Geometry: final body of the model. Coordinates: model frame, mm. A direction names the side the tool comes from. Give positions to 0.01 mm unless a question says otherwise; leave off trailing zeros. Loops run counter-clockwise (first coordinate to the right, second up) from the corner with the lowest first, then second, coordinate; pieces in that order, holes last. Notation, with made-up numbers: (-36, -26) -> (-20, -26) arc R23 cw to (-20, -5) -> close; hole circle Ø6 at (-28.75, 86). An arc over 180 degrees is marked (long way). One line per item, written item: value. Start each with the question number.
from build123d import *

# Parameters (mm, degrees)
F_4_5_4_5_DIAMETER_HOLE1_D = 4.5
CIRPATTERN1_COUNT          = 12
F_4_0_4_DIAMETER_HOLE1_D   = 4
CIRPATTERN2_COUNT          = 4
CIRPATTERN3_COUNT          = 4


with BuildPart() as part:
    # Sketch1 → Revolve1 (revolve)
    with BuildSketch(Plane(origin=(0, 0, 0), x_dir=(0, 0, -1), z_dir=(1, 0, 0)), mode=Mode.PRIVATE) as revolve1_sk:
        with BuildLine():
            Line((0, 129), (0, 121.95))
            ThreePointArc((0, 121.95), (-0.878679656, 119.828679656), (-3, 118.95))
            Line((-3, 118.95), (-28, 118.95))
            Line((-28, 118.95), (-28, 119.95))
            Line((-28, 119.95), (-3, 119.95))
            ThreePointArc((-3, 119.95), (-1.585786438, 120.535786438), (-1, 121.95))
            Line((-1, 121.95), (-1, 129))
            Line((-1, 129), (0, 129))
        make_face()
    revolve(revolve1_sk.sketch.rotate(Axis((0, 0, 36.289125048), (0, 0, -1)), 90), axis=Axis((0, 0, 36.289125048), (0, 0, -1)))  # turned: the seam where the file's is

    # Ø4.5 (4.5) Diameter Hole1 (through all)
    with Locations(Plane.XY.offset(1)):
        with Locations((62.125, 107.60365642)):
            f_4_5_4_5_diameter_hole1 = Hole(F_4_5_4_5_DIAMETER_HOLE1_D / 2)

    # CirPattern1: Ø4.5 (4.5) Diameter Hole1 ×12 about axis, 4 skipped
    cirpattern1_axis = Axis((0, 0, -80.9), (0, 0, 1))
    add([f_4_5_4_5_diameter_hole1.rotate(cirpattern1_axis, i * 360 / CIRPATTERN1_COUNT) for i in range(1, CIRPATTERN1_COUNT) if i not in (1, 4, 7, 10)], mode=Mode.SUBTRACT)

    # Ø4.0 (4) Diameter Hole1 (through all)
    with Locations(Plane.XY.offset(1)):
        with Locations((124.25, 0)):
            f_4_0_4_diameter_hole1 = Hole(F_4_0_4_DIAMETER_HOLE1_D / 2)

    # CirPattern2: Ø4.0 (4) Diameter Hole1 ×4 about axis
    cirpattern2_axis = Axis((0, 0, 0), (0, 0, 1))
    for i in range(1, CIRPATTERN2_COUNT):
        add(f_4_0_4_diameter_hole1.rotate(cirpattern2_axis, i * 360 / CIRPATTERN2_COUNT), mode=Mode.SUBTRACT)

    # Sketch7 → Ø4.5 (4.5) Diameter Hole2 (revolve, cut)
    with BuildSketch(Plane(origin=(87.858017562, 87.858017562, 1), x_dir=(0, -1, 0), z_dir=(1, 0, 0))):
        Polygon((0, 0), (0, 2.851936393), (2.25, 1.5), (2.25, 0), align=None)
    f_4_5_4_5_diameter_hole2 = revolve(axis=Axis((87.858017562, 87.858017562, 7.35), (0, 0, -1)), mode=Mode.SUBTRACT)

    # CirPattern3: Ø4.5 (4.5) Diameter Hole2 ×4 about axis
    cirpattern3_axis = Axis((0, 0, 0), (0, 0, 1))
    for i in range(1, CIRPATTERN3_COUNT):
        add(f_4_5_4_5_diameter_hole2.rotate(cirpattern3_axis, i * 360 / CIRPATTERN3_COUNT), mode=Mode.SUBTRACT)


solid = part.part
Item 1: Pin query (flat end, axial travel): pin 1 (6 mm diameter, centred on y = 17.5, z = 10.5, fed in from -X); pin 2 (6 mm diameter, centred on x = 87.86, y = -87.86, fed in from +Z); pin 3 (3.5 mm diameter, centred on x = -62.12, y = 107.6, fed in from +Z); pin 4 (4 mm diameter, centred on x = -82.5, z = 25, fed in from +Y). Return the tip coordinate at first contact, or that it passes through.
Item 2: Mould query, pull axis Y, two halves, no side actions, for faces 3 (the face through (113.457, -35.729, 15.675)), 4 (the face through (123.043, -38.748, 0.493)), 5 (the face through (116, -27, 28)). Classes: pulls with the +Y half, pulls with the -Y half, needs draft (parallel to the pull), parting line crosses it, or undercut.
Item 3: Ray query, line 1 along X through (y, z) = (-68, 26); line 2 along Y through (x, z) = (66.5, 6); line 3 along Y through (x, z) = (-32, 2). Return the intervals inside material, ascending. Write a range as [from, to].
Item 4: Access query for faces 1 (the face through (47, 114, 0)), 2 (the face through (-114, 47, 1)). Directions: +Z, -Z, +X, -X, +Y, -Y. A direction counts if a zero-diameter tool reaches every point of the face in a straight line with its end or side. Return the directions, or none.
Item 5: Section A-A, the plane z = 20.5. Output: boundary loops of the cut face in (x, y).
Geometry check:
1. pin 1: stops at x = -119.07
1. pin 2: stops at z = 1.13
1. pin 3: passes through
1. pin 4: stops at y = 88.93
2. face 3: undercut
2. face 4: parting line crosses it
2. face 5: needs draft
3. line 1: x = [-98.81, -97.6], [97.6, 98.81]
3. line 2: y = [-99.83, -98.62], [98.62, 99.83]
3. line 3: y = [-115.88, -114.74], [114.74, 115.88]
4. face 1: -Z, +X, -X, +Y, -Y
4. face 2: +Z
5. outline: circle Ø239.9 at (0, 0); hole circle Ø237.9 at (0, 0)
